Verification items for this drawing (mm, ordinates from the low corner). A direction names the side the tool comes from. Give positions to 0.01 mm unless a question says otherwise; leave off trailing zeros. Order: outer loops, then holes, each group sorted by start corner. A loop starts at its lowest first (then second) coordinate and runs counter-clockwise, first axis right, second up. Notation, with made-up numbers: M 0,-13.5 L 47,-13.5 A18 ccw 47,10.5 Z; hole C 8,2.5 d3. An arc over 180 degrees is marked long. Answer as a JSON object with one key per item and string values.
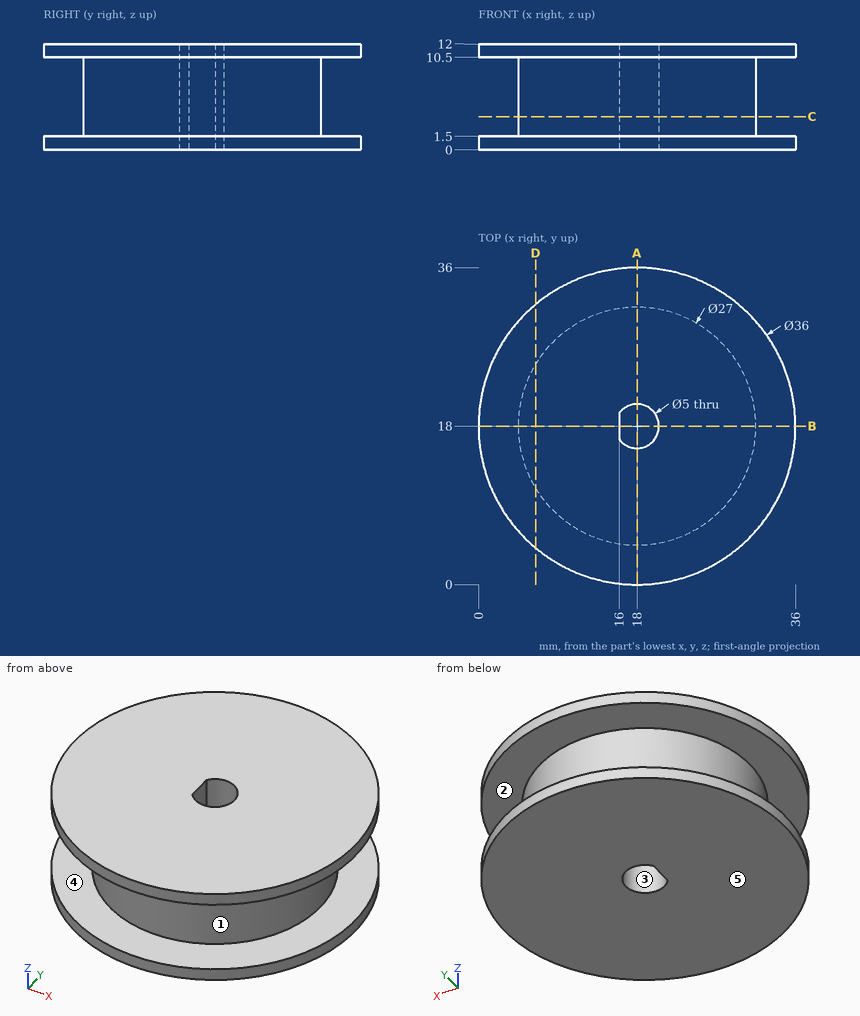
Q1. Section check A-A on x = 18. Record the cut outline in (y, z), then the cut area to 3 significant figures.
Resolved:
{"outline": "M 0,0 L 15.5,0 L 15.5,12 L 0,12 L 0,10.5 L 4.5,10.5 L 4.5,1.5 L 0,1.5 Z; M 20.5,0 L 36,0 L 36,1.5 L 31.5,1.5 L 31.5,10.5 L 36,10.5 L 36,12 L 20.5,12 Z", "area": "291 mm²"}
Q2. Release check for a two-part mould opening along X. For the marked faces 1, 2 and 3 record: +X half, -X half, draft (parallel to the pull), parting line (faces both ways), or undercut.
Resolved:
{"face 1": "parting line", "face 2": "draft", "face 3": "undercut"}
Q3. Material ranges on L1, parallel to Z at x = 4, y = 18.5; L2, parallel to X at y = 18, z = 4.75; L3, parallel to X at y = 18, z = 11, recorded low to high.
Resolved:
{"L1": "z = 0 to 1.5, 10.5 to 12", "L2": "x = 4.5 to 16, 20.5 to 31.5", "L3": "x = 0 to 16, 20.5 to 36"}
Q4. Section check B-B on y = 18. Record the cut outline in (x, z), then the cut area to 3 significant figures.
Resolved:
{"outline": "M 0,0 L 16,0 L 16,12 L 0,12 L 0,10.5 L 4.5,10.5 L 4.5,1.5 L 0,1.5 Z; M 20.5,0 L 36,0 L 36,1.5 L 31.5,1.5 L 31.5,10.5 L 36,10.5 L 36,12 L 20.5,12 Z", "area": "297 mm²"}
Q5. Section check C-C on z = 3.75. Record the cut outline in (x, y).
Resolved:
{"outline": "C 18,18 d27; hole M 16,16.5 A2.5 ccw long 16,19.5 Z"}
Q6. Tool access check on the marked faces 4 and 5. Record the directions out of +Z, -Z, +X, -X, +Y, -Y that give a thin tool (end or side, any length) a straight path to the whole face; none if there is none.
Resolved:
{"face 4": "none", "face 5": "-Z, +X, -X, +Y, -Y"}
Q7. Section check D-D on x = 6.5. Record the cut outline in (y, z).
Resolved:
{"outline": "M 4.15,0 L 31.85,0 L 31.85,1.5 L 25.07,1.5 L 25.07,10.5 L 31.85,10.5 L 31.85,12 L 4.15,12 L 4.15,10.5 L 10.93,10.5 L 10.93,1.5 L 4.15,1.5 Z"}
Q8. Gauge pin test, flat ends, axial feed: pin 1 Ø1 at (x, y) = (23, 24) entering from -Z; pin 2 Ø4 at (x, z) = (5, 3) entering from +Y; pin 3 Ø1 at (x, z) = (11, 6) entering from -Y; pin 4 Ø1.5 at (y, z) = (17.5, 6) entering from +X. Record the tip position at first contact, or that the pin passes through.
Resolved:
{"pin 1": "stops at z = 0", "pin 2": "stops at y = 31.7", "pin 3": "stops at y = 6.17", "pin 4": "stops at x = 31.5"}
